Build history of the part. All positions in model axes, mm. A direction names the side the tool comes from. Round coordinates to 2 decimals unless told otherwise and drop trailing zeros. Write each loop counter-clockwise with the first axis right and the second up, starting at its lowest first coordinate (ties: lowest second). Pieces come first, ordered by that corner, then holes.
Item 1: Band-saw the part on A-A, the plane x = 43.5. Write the cut outline in (y, z).
Item 2: Band-saw the part on B-B, the plane y = 12.5. Write the cut outline in (x, z).
Item 3: Band-saw the part on C-C, the plane z = 9. Write the cut outline in (x, y) (3 decimals), then the cut area to 3 significant figures.
Item 4: 3-axis set-ups, long thin cutter, end or side, ignore diameter. For faces 1 (the cylindrical face through (53.592, 2.487, -23.792)), 2 (the cylindrical face through (2.49, 2.54, -23.79)), 3 (the cylindrical face through (27.379, 24.968, 16.504)): which of +Z, -Z, +X, -X, +Y, -Y reach the whole face in a straight line?
Item 5: Drop flat-ended pins along their axis: pin 1 Ø10 at (x, y) = (16, 11) entering from +Z; pin 2 Ø3 at (x, y) = (1.5, 1.5) entering from -Z; pin 3 Ø1.1 at (x, y) = (1, 54.5) entering from -Z. Give the stop position or say it passes through.
Item 6: Wall check: probe 1 along Z at (x, y) = (35.5, 44); probe 2 along Z at (x, y) = (49, 32.5); probe 3 along Y at (x, z) = (54, -34). Give the ranges that are in metal, low to high.
Item 7: Band-saw the part on D-D, the plane y = 29.5. Write the cut outline in (x, z), then the cut area to 3 significant figures.
```python
from build123d import *

# Parameters (mm, degrees)
SKETCH2_W           = 56.134
SKETCH2_H           = 56.134
BOSS_EXTRUDE1_DEPTH = 5.461
SKETCH3_R           = 19.05
BOSS_EXTRUDE2_DEPTH = 1.651
BOSS_EXTRUDE3_DEPTH = 48.26
SKETCH5_R           = 3.175
BOSS_EXTRUDE4_DEPTH = 19.05


with BuildPart() as part:
    # Sketch2 → Boss-Extrude1 (new body)
    with BuildSketch(Plane.XY):
        with Locations((28.067, 28.067)):
            Rectangle(SKETCH2_W, SKETCH2_H)
    extrude(amount=BOSS_EXTRUDE1_DEPTH)

    # Sketch3 → Boss-Extrude2 (add)
    with BuildSketch(Plane.XY.offset(5.461)):
        with Locations((28.067, 28.067)):
            Circle(SKETCH3_R)
    extrude(amount=BOSS_EXTRUDE2_DEPTH)

    # Sketch4 → Boss-Extrude3 (add)
    with BuildSketch(Plane(origin=(0, 0, 0), x_dir=(-1, 0, 0), z_dir=(0, 0, -1))):
        with BuildLine():
            Line((-52.578, 56.134), (-3.556, 56.134))
            ThreePointArc((-3.556, 56.134), (-2.514471714, 53.619528286), (0, 52.578))
            Line((0, 52.578), (0, 3.556))
            ThreePointArc((0, 3.556), (-2.514471714, 2.514471714), (-3.556, 0))
            Line((-3.556, 0), (-52.578, 0))
            ThreePointArc((-52.578, 0), (-53.619528286, 2.514471714), (-56.134, 3.556))
            Line((-56.134, 3.556), (-56.134, 52.578))
            ThreePointArc((-56.134, 52.578), (-53.619528286, 53.619528286), (-52.578, 56.134))
        make_face()
    extrude(amount=BOSS_EXTRUDE3_DEPTH)

    # Sketch5 → Boss-Extrude4 (add)
    with BuildSketch(Plane.XY.offset(7.112)):
        with Locations((28.067, 28.067)):
            Circle(SKETCH5_R)
    extrude(amount=BOSS_EXTRUDE4_DEPTH)


solid = part.part
```
Results:
1. outline: (0, -48.26) - (56.13, -48.26) - (56.13, 5.46) - (39.24, 5.46) - (39.24, 7.11) - (16.9, 7.11) - (16.9, 5.46) - (0, 5.46) - close
2. outline: (0, -48.26) - (56.13, -48.26) - (56.13, 5.46) - (39.05, 5.46) - (39.05, 7.11) - (17.09, 7.11) - (17.09, 5.46) - (0, 5.46) - close
3. outline: circle Ø6.35 at (28.067, 28.067)
3. area: 31.7 mm2
4. face 1: -Z, +X, -Y
4. face 2: -Z, -X, -Y
4. face 3: +Z
5. pin 1: stops at z = 7.11
5. pin 2: stops at z = -48.26
5. pin 3: stops at z = 0
6. probe 1: z = -48.26 to 7.11
6. probe 2: z = -48.26 to 5.46
6. probe 3: y = 2.84 to 53.29
7. outline: (0, -48.26) - (56.13, -48.26) - (56.13, 5.46) - (47.06, 5.46) - (47.06, 7.11) - (30.9, 7.11) - (30.9, 26.16) - (25.23, 26.16) - (25.23, 7.11) - (9.07, 7.11) - (9.07, 5.46) - (0, 5.46) - close
7. area: 3,190 mm2
